The listing builds one solid part. Answer for the finished solid, in the listing's coordinates (mm). Face numbers are marked on the shaded views. A direction names the side the tool comes from. Coordinates: 2 decimals unless noted, no trailing zeros. Loops run counter-clockwise (first coordinate to the right, second up) from the corner with the lowest first, then second, coordinate; pieces in that order, holes last. Notation, with made-up numbers: (-15.75, 83.5) - (41.25, 83.5) arc R16 ccw to (41.25, 93.5) - close; hole circle Ø9 at (64, -5). An arc over 180 degrees is marked (long way). Write each question's results on one line, items separated by ' | '. Start each with the question number.
(1) Find section A-A on y = 29. Determine the outline of the cut face in (x, z), then the cut area to 3 significant figures.
(2) Given pin 1 Ø4 at (x, z) = (0, 43.5) entering from +Y; pin 2 Ø8 at (x, z) = (-15, 27.5) entering from +Y, each flat-ended and moving along its own axis, determine where each tip first touches the part or whether it passes through.
(3) Find section B-B on z = 43.5. Determine the outline of the cut face in (x, y), then the cut area to 3 significant figures.
(4) Find section D-D on x = 0. Determine the outline of the cut face in (y, z).
(5) Determine the mould class of the marked faces 1, 2 and 3 for opening direction X: released by +X, released by -X, zero draft, split by the parting line, or undercut.
(6) Consider line 1 (X direction, y = 28, z = 45); line 2 (Y direction, x = -12.5, z = 26); line 3 (X direction, y = 19, z = 24.5). Determine where each line is inside the solid, lowest interval first. Write a range as from..to.
(7) For the marked faces 4 and 5, determine the directions among +Z, -Z, +X, -X, +Y, -Y from which every point of the face is accessible in a straight line to the end or side of a thin tool.
(8) Find section C-C on x = -14. Determine the outline of the cut face in (y, z), then the cut area to 3 significant figures.
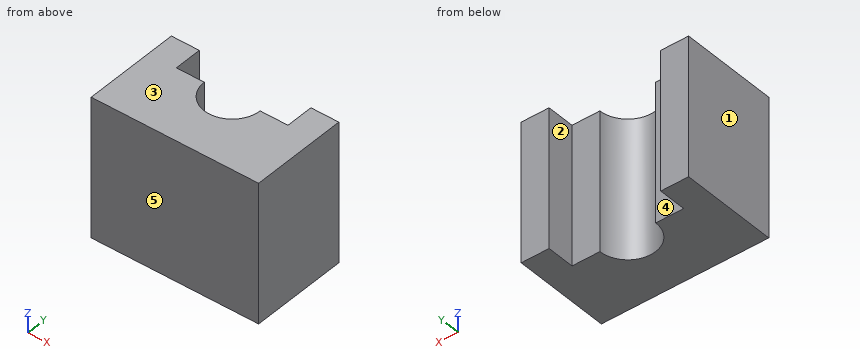
from build123d import *

# Parameters (mm, degrees)
BOSS_EXTRUDE1_DEPTH = 50


with BuildPart() as part:
    # Sketch1 → Boss-Extrude1 (new body)
    with BuildSketch(Plane.XY):
        with BuildLine():
            Line((-20, 35), (-20, 25))
            Line((-20, 25), (-10, 25))
            ThreePointArc((-10, 25), (0, 15), (10, 25))
            Line((10, 25), (20, 25))
            Line((20, 25), (20, 35))
            Line((20, 35), (30, 35))
            Line((30, 35), (30, 0))
            Line((30, 0), (-30, 0))
            Line((-30, 0), (-30, 35))
            Line((-30, 35), (-20, 35))
        make_face()
    extrude(amount=BOSS_EXTRUDE1_DEPTH)


solid = part.part
Values:
1) outline: (-30, 0) - (-20, 0) - (-20, 50) - (-30, 50) - close; (20, 0) - (30, 0) - (30, 50) - (20, 50) - close | area: 1,000 mm²
2) pin 1: stops at y = 15.2 | pin 2: stops at y = 25
3) outline: (-30, 0) - (30, 0) - (30, 35) - (20, 35) - (20, 25) - (10, 25) arc R10 cw to (-10, 25) - (-20, 25) - (-20, 35) - (-30, 35) - close | area: 1,540 mm²
4) outline: (0, 0) - (15, 0) - (15, 50) - (0, 50) - close
5) face 1: released by -X | face 2: undercut | face 3: zero draft
6) line 1: x = -30..-20, 20..30 | line 2: y = 0..25 | line 3: x = -30..-8, 8..30
7) face 4: +Z, -Z, +Y | face 5: +Z, -Z, +X, -X, -Y
8) outline: (0, 0) - (25, 0) - (25, 50) - (0, 50) - close | area: 1,250 mm²
